Can you work these out from the drawing? Everything is in mm from the part's minimum corner. A direction names the side the tool comes from. Round coordinates to 2 decimals unless told otherwise and drop trailing zeros. Loops run counter-clockwise (first coordinate to the right, second up) from the corner with the lowest first, then second, coordinate; pieces in that order, holes last. Notation, with made-up numbers: M 77.25,17.5 L 102.25,17.5 A14 ccw 102.25,41.5 Z; hole C 45.25,-28.75 d9. An arc over 180 degrees is marked long. Answer in a Markdown table with one row per item.
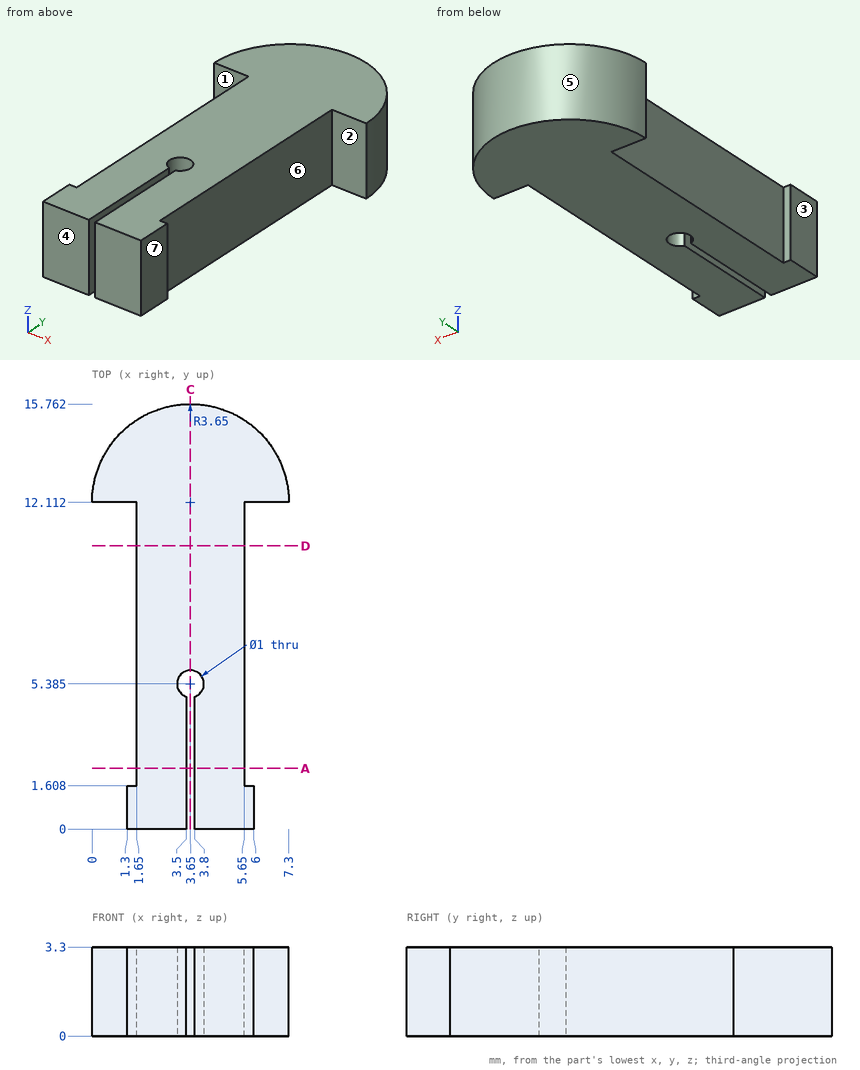
1) I want a section at C-C, the plane x = 3.65. Please give me the cut outline in (y, z) (1 decimal).
Computed:
| item | result |
|---|---|
| outline | M 5.9,0 L 15.8,0 L 15.8,3.3 L 5.9,3.3 Z |
2) Which directions (+Z, -Z, +X, -X, +Y, -Y) give clear straight access to the entire face, cutting with the end or side of a thin tool? Please do the marked faces 1, 2 and 3.
Computed:
| item | result |
|---|---|
| face 1 | +Z, -Z, -X |
| face 2 | +Z, -Z, +X |
| face 3 | +Z, -Z, -X, -Y |
3) If we mould it in two halves opening along Y, with no side actions, what happens to the marked faces 4, 5, 6 and 7? For each: released by +Y, released by -Y, zero draft, split by the parting line, or undercut.
Computed:
| item | result |
|---|---|
| face 4 | released by -Y |
| face 5 | released by +Y |
| face 6 | undercut |
| face 7 | zero draft |
4) I need wall thicknesses on line 1 (X direction, y = 4.5, z = 2.2); line 2 (X direction, y = 1, z = 1.4); line 3 (Y direction, x = 3.65, z = 0.7) (1 decimal). Which ranges of each line are inside material? Lowest first, please.
Computed:
| item | result |
|---|---|
| line 1 | x = 1.65 to 3.5, 3.8 to 5.65 |
| line 2 | x = 1.3 to 3.5, 3.8 to 6 |
| line 3 | y = 5.9 to 15.8 |
5) Will these pins go through, and if not, where does the flat tip stop? P1, Ø1.3, axis at y = 1, z = 1, coming from the -X side; P2, Ø1.8, axis at y = 1, z = 2, coming from the +X side; P3, Ø0.5, axis at x = 0.5, z = 1, coming from the -Y side; P4, Ø0.8, axis at x = 6, z = 2, coming from the -Y side.
Computed:
| item | result |
|---|---|
| P1 | stops at x = 1.3 |
| P2 | stops at x = 6 |
| P3 | stops at y = 12.11 |
| P4 | stops at y = 0 |
6) I want a section at A-A, the plane y = 2.25. Please give me the cut outline in (x, z), plus the area to 3 significant figures.
Computed:
| item | result |
|---|---|
| outline | M 1.65,0 L 3.5,0 L 3.5,3.3 L 1.65,3.3 Z; M 3.8,0 L 5.65,0 L 5.65,3.3 L 3.8,3.3 Z |
| area | 12.2 mm² |
7) I want a section at D-D, the plane y = 10.5. Please give me the cut outline in (x, z).
Computed:
| item | result |
|---|---|
| outline | M 1.65,0 L 5.65,0 L 5.65,3.3 L 1.65,3.3 Z |
